Can you work these out from the model? Positions are in its coordinate system, mm. A direction names the side the tool comes from. Coordinates: 2 decimals unless noted, no trailing zeros. Loops run counter-clockwise (first coordinate to the right, second up) from the corner with the lowest first, then second, coordinate; pieces in that order, holes last.
```python
from build123d import *

# Parameters (mm, degrees)
SKETCH1_W                      = 15.24
SKETCH1_H                      = 13.97
BOSS_EXTRUDE1_DEPTH            = 5.08
SKETCH2_W                      = 15.24
SKETCH2_H                      = 5.08
BOSS_EXTRUDE2_DEPTH            = 9.652
M3_CLEARANCE_HOLE1_D           = 3.7
M3_CLEARANCE_HOLE1_DEPTH       = 25.4
M3_CLEARANCE_HOLE1_TIP         = 1.111592145
CBORE_FOR_M3_SHCS2_D           = 3.6
CBORE_FOR_M3_SHCS2_DEPTH       = 25.4
CBORE_FOR_M3_SHCS2_CBORE_D     = 6.5
CBORE_FOR_M3_SHCS2_CBORE_DEPTH = 3
CBORE_FOR_M3_SHCS2_TIP         = 1.081549114


with BuildPart() as part:
    # Sketch1 → Boss-Extrude1 (new body)
    with BuildSketch(Plane(origin=(0, 0, 0), x_dir=(1, 0, 0), z_dir=(0, 1, 0))):
        with Locations((0.762, 3.81)):
            Rectangle(SKETCH1_W, SKETCH1_H)
    extrude(amount=BOSS_EXTRUDE1_DEPTH)

    # Sketch2 → Boss-Extrude2 (add)
    with BuildSketch(Plane(origin=(0, 5.08, 0), x_dir=(1, 0, 0), z_dir=(0, 1, 0))):
        with Locations((0.762, 8.255)):
            Rectangle(SKETCH2_W, SKETCH2_H)
    extrude(amount=BOSS_EXTRUDE2_DEPTH)

    # M3 Clearance Hole1
    with Locations(Plane.XY.offset(-5.715)):
        with Locations((0.762, 8.89)):
            Hole(M3_CLEARANCE_HOLE1_D / 2, depth=M3_CLEARANCE_HOLE1_DEPTH)
            with Locations((0, 0, -(M3_CLEARANCE_HOLE1_DEPTH + M3_CLEARANCE_HOLE1_TIP / 2))):  # 118° drill point
                Cone(0, M3_CLEARANCE_HOLE1_D / 2, M3_CLEARANCE_HOLE1_TIP, mode=Mode.SUBTRACT)

    # CBORE for M3 SHCS2
    with Locations(Plane(origin=(0, 5.08, 0), x_dir=(1, 0, 0), z_dir=(0, 1, 0))):
        with Locations((0.762, 1.905)):
            CounterBoreHole(CBORE_FOR_M3_SHCS2_D / 2, CBORE_FOR_M3_SHCS2_CBORE_D / 2, CBORE_FOR_M3_SHCS2_CBORE_DEPTH, depth=CBORE_FOR_M3_SHCS2_DEPTH)
            with Locations((0, 0, -(CBORE_FOR_M3_SHCS2_DEPTH + CBORE_FOR_M3_SHCS2_TIP / 2))):  # 118° drill point
                Cone(0, CBORE_FOR_M3_SHCS2_D / 2, CBORE_FOR_M3_SHCS2_TIP, mode=Mode.SUBTRACT)


solid = part.part
```
(1) If we mould it in two halves opening along Y, with no side actions, what happens to faces 1 (the flat face through (1, 14.732, -8)), 2 (the flat face through (1, 11, -5.715)), 3 (the cylindrical face through (1.163, 7.084, -8.291))? For each: released by +Y, released by -Y, zero draft, split by the parting line, or undercut.
Check values:
face 1: released by +Y
face 2: zero draft
face 3: undercut
(2) If I drill on probe 1 along Z at (x, y) = (3.75, 11) (3 decimals); probe 2 along Y at (x, z) = (5.25, 0.25); probe 3 along Y at (x, z) = (1.5, -9), over which ranges is the centre line in solid material (lowest first)?
Check values:
probe 1: z = -10.795 to -5.715
probe 2: y = 0 to 5.08
probe 3: y = 0 to 7.19, 10.59 to 14.73
(3) Which directions (+Z, -Z, +X, -X, +Y, -Y) give clear straight access to the entire face, cutting with the end or side of a thin tool? Please do faces 4 (the flat face through (1, 0, -4)), 5 (the flat face through (1, 5.08, 2)), 6 (the cylindrical face through (-1.82, 3.6, 0.07)).
Check values:
face 4: +Z, -Z, +X, -X, -Y
face 5: +Z, +X, -X, +Y
face 6: +Y
(4) I want a section at B-B on x = 1.25. Write out the boundary of the cut face in (y, z) (3 decimals), then the cut area to 3 significant figures.
Check values:
outline: (0, -10.795) - (7.106, -10.795) - (7.106, -5.715) - (5.08, -5.715) - (5.08, -5.118) - (2.08, -5.118) - (2.08, -3.638) - (0, -3.638) - close; (0, -0.172) - (2.08, -0.172) - (2.08, 1.308) - (5.08, 1.308) - (5.08, 3.175) - (0, 3.175) - close; (10.674, -10.795) - (14.732, -10.795) - (14.732, -5.715) - (10.674, -5.715) - close
area: 75.4 mm2
(5) I want a section at D-D on z = 0.5. Write out the boundary of the cut face in (x, y).
Check values:
outline: (-6.86, 0) - (8.38, 0) - (8.38, 5.08) - (2.95, 5.08) - (2.95, 2.08) - (-1.42, 2.08) - (-1.42, 5.08) - (-6.86, 5.08) - close
(6) I want a section at C-C on z = -8. Write out the boundary of the cut face in (x, y).
Check values:
outline: (-6.86, 0) - (8.38, 0) - (8.38, 14.73) - (-6.86, 14.73) - close; hole circle Ø3.7 at (0.76, 8.89)
(7) I'm going to push flat-ended pins straight in: pin 1 (2 mm diameter, centred on x = 0.762, z = -1.905, fed in from -Y); pin 2 (7.5 mm diameter, centred on x = 0.762, z = -1.905, fed in from +Y); pin 3 (2.5 mm diameter, centred on x = 1, z = -3, fed in from +Y); pin 4 (1.5 mm diameter, centred on x = 7, y = 6, fed in from +Z) (3 decimals). Where does each tip first touch, or does it pass through?
Check values:
pin 1: passes through
pin 2: stops at y = 5.08
pin 3: stops at y = 2.08
pin 4: stops at z = -5.715
(8) I want a section at A-A on y = 8.89. Write out the boundary of the cut face in (x, z) (3 decimals), then the cut area to 3 significant figures.
Check values:
outline: (-6.858, -10.795) - (-1.088, -10.795) - (-1.088, -5.715) - (-6.858, -5.715) - close; (2.612, -10.795) - (8.382, -10.795) - (8.382, -5.715) - (2.612, -5.715) - close
area: 58.6 mm2
